from build123d import *

# Parameters (mm, degrees)
F2_SIZE = 1.8
F3_SIZE = 0.3
F4_SIZE = 0.2


with BuildPart() as f1:
    # F0 (on Top) → F1 (revolve)
    with BuildSketch(Plane.XY):
        Polygon((-2, 7.1), (0, 7.1), (0, 8.25), (2, 8.25), (2, 10.75), (-2, 10.75), align=None)
    revolve(axis=Axis((-1, 0, 0), (-1, 0, 0)))

    # F2
    f2_edges = [f1.edges().sort_by_distance(p)[0] for p in [
        (-2, -10.75, 0),
    ]]
    chamfer(f2_edges, length=F2_SIZE)

    # F3
    f3_edges = [f1.edges().sort_by_distance(p)[0] for p in [
        (-2, -7.1, 0),
    ]]
    chamfer(f3_edges, length=F3_SIZE)

    # F4
    f4_edges = [f1.edges().sort_by_distance(p)[0] for p in [
        (2, -8.25, 0),
        (0, -7.1, 0),
    ]]
    chamfer(f4_edges, length=F4_SIZE)


solid = f1.part
Read the model definition and answer for the solid it produces. Units are mm, in the model's axes. A direction names the side the tool comes from. Give positions to 0.01 mm unless a question says otherwise; leave off trailing zeros. Write each loop counter-clockwise with the first axis right and the second up, starting at its lowest first coordinate (ties: lowest second). Pieces come first, ordered by that corner, then holes. Notation, with made-up numbers: (10, 16) - (28, 16) arc R10 ccw to (28, 26) - close; hole circle Ø3 at (45.25, 31). An arc over 180 degrees is marked (long way). Use CSV: the item, a comma, the result in double quotes. Start each with the question number.
Item 1: Consider line 1 (Y direction, x = 0.6, z = 0); line 2 (Z direction, x = -0.95, y = -3.75). Determine where each line is inside the solid, lowest interval first.
Item 2: The part is cut by section A-A, the plane z = 0. Give the vertices of the cut face in (x, y).
Item 3: For faces 1 (the cylindrical face through (0.91, 7.62, 3.16)), 2 (the flat face through (-2, -3, -7)), determine the directions among +Z, -Z, +X, -X, +Y, -Y from which every point of the face is accessible in a straight line to the end or side of a thin tool.
Item 4: The mould has two halves that part along Y. Classify faces 3 (the cylindrical face through (0.88, -1.4, -10.66)), 4 (the flat face through (2, -5, 7)), 5 (the cylindrical face through (-0.94, -0.92, -7.04)): pulls with the +Y half, pulls with the -Y half, needs draft (parallel to the pull), parting line crosses it, or undercut.
Item 5: The part is cut by section C-C, the plane x = 1.1. Give the vertices of the cut face in (y, z).
Taken from the geometry:
1,line 1,"-10.75 to -8.25, 8.25 to 10.75"
1,line 2,"-9.27 to -6.03, 6.03 to 9.27"
2,outline,"(-2, -8.95) - (-0.2, -10.75) - (2, -10.75) - (2, -8.45) - (1.8, -8.25) - (0, -8.25) - (0, -7.3) - (-0.2, -7.1) - (-1.7, -7.1) - (-2, -7.4) - close; (-2, 7.4) - (-1.7, 7.1) - (-0.2, 7.1) - (0, 7.3) - (0, 8.25) - (1.8, 8.25) - (2, 8.45) - (2, 10.75) - (-0.2, 10.75) - (-2, 8.95) - close"
3,face 1,"+X"
3,face 2,"+Z, -Z, -X, +Y, -Y"
4,face 3,"parting line crosses it"
4,face 4,"needs draft"
4,face 5,"undercut"
5,outline,"circle Ø21.5 at (0, 0); hole circle Ø16.5 at (0, 0)"
